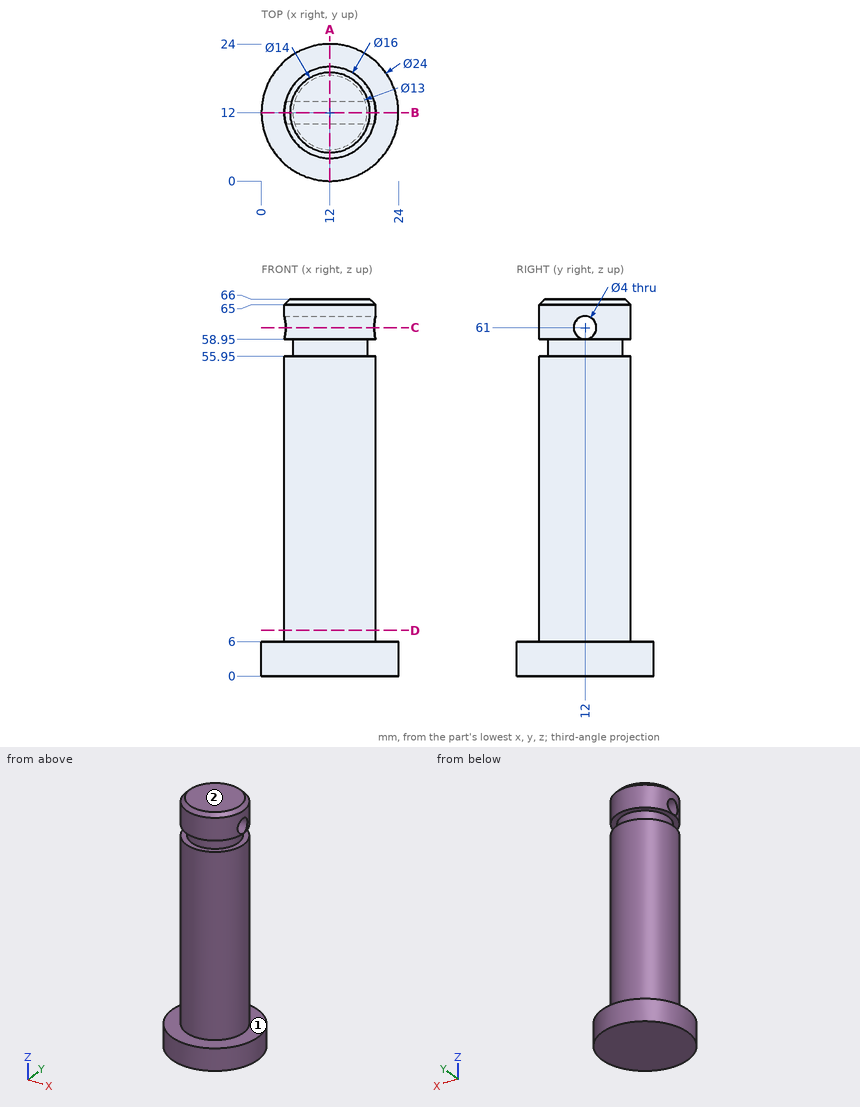
Geometry: see drawing. Coordinates: mm, zero at the bounding-box minimum. A direction names the side the tool comes from. Give positions to 0.01 mm unless a question says otherwise; leave off trailing zeros. Write each loop counter-clockwise with the first axis right and the second up, starting at its lowest first coordinate (ties: lowest second). Pieces come first, ordered by that corner, then holes. Notation, with made-up numbers: (69, 12) - (124, 12) arc R34 cw to (124, 48) - close; hole circle Ø11 at (81.5, 18.5). An arc over 180 degrees is marked (long way). Return JSON: item names as keys, results as strings. Group by question number.
1) Line query: line 1 (Z direction, x = 11.25, y = 12); line 2 (Y direction, x = 12, z = 45.5); line 3 (Z direction, x = 16.5, y = 17.75). Output: solid intervals per line, ascending.
2) Section A-A on x = 12. Return the cut outline in (y, z), plus the area to 3 significant figures.
3) Section C-C on z = 61. Return the cut outline in (x, y), plus the area to 3 significant figures.
4) Set-up query: the marked faces 1 and 2. Return all of +Z, -Z, +X, -X, +Y, -Y with unobstructed straight access to the full face (end or side cutting, diameter ignored); none if empty.
5) Section B-B on y = 12. Return the cut outline in (x, z), plus the area to 3 significant figures.
6) Section D-D on z = 8. Return the cut outline in (x, y).
7) First-contact query: P1, Ø6, axis at x = 19, z = 26, coming from the -Y side; P2, Ø12, axis at x = 8.5, z = 50, coming from the -Y side; P3, Ø1, axis at x = 8, z = 17.5, coming from the +Y side; P4, Ø2.5, axis at y = 12, z = 61, coming from the +X side. Flat tips, straight axial feed; report the tip coordinate or a pass-through.
Filled in:
{
 "1": {"line 1": "z = 0 to 59, 63 to 66", "line 2": "y = 4 to 20", "line 3": "z = 0 to 55.95, 58.95 to 65.7"},
 "2": {"outline": "(0, 0) - (24, 0) - (24, 6) - (20, 6) - (20, 55.95) - (18.5, 55.95) - (18.5, 58.95) - (20, 58.95) - (20, 65) - (19, 66) - (5, 66) - (4, 65) - (4, 58.95) - (5.5, 58.95) - (5.5, 55.95) - (4, 55.95) - (4, 6) - (0, 6) - close; hole circle Ø4 at (12, 61)", "area": "1,080 mm^2"},
 "3": {"outline": "(4.25, 10) arc R8 ccw to (19.75, 10) - close; (4.25, 14) - (19.75, 14) arc R8 ccw to start", "area": "138 mm^2"},
 "4": {"face 1": "+Z", "face 2": "+Z, +X, -X, +Y, -Y"},
 "5": {"outline": "(0, 0) - (24, 0) - (24, 6) - (20, 6) - (20, 55.95) - (18.5, 55.95) - (18.5, 58.95) - (20, 58.95) - (20, 59) - (4, 59) - (4, 58.95) - (5.5, 58.95) - (5.5, 55.95) - (4, 55.95) - (4, 6) - (0, 6) - close; (4, 63) - (20, 63) - (20, 65) - (19, 66) - (5, 66) - (4, 65) - close", "area": "1,030 mm^2"},
 "6": {"outline": "circle Ø16 at (12, 12)"},
 "7": {"P1": "stops at y = 5.07", "P2": "stops at y = 4", "P3": "stops at y = 19.19", "P4": "passes through"}
}
